```python
from build123d import *


with BuildPart() as part:
    # Sketch1 → Revolve1 (revolve)
    with BuildSketch(Plane.XY):
        with BuildLine():
            Line((0, 0), (0, 7.14024037))
            ThreePointArc((0, 7.14024037), (-10.863552097, 19.485230229), (-24.489599009, 10.279450287))
            ThreePointArc((-24.489599009, 10.279450287), (-27.821731607, 7.348582007), (-31.501935722, 9.82833889))
            ThreePointArc((-31.501935722, 9.82833889), (-35.138176859, 13.576179652), (-40.254364407, 12.530624802))
            ThreePointArc((-40.254364407, 12.530624802), (-42.51580515, 12.328830241), (-44.6786, 13.019593379))
            Line((-44.6786, 13.019593379), (-45.466, 13.019593379))
            Line((-45.466, 13.019593379), (-45.466, 0))
            Line((-45.466, 0), (0, 0))
        make_face()
    revolve(axis=Axis((-45.466, 0, 0), (0, 1, 0)))


solid = part.part
```
CAD build for the part. Positions are in the model's coordinates, mm. Coordinates: 2 decimals unless noted, no trailing zeros. Order: outer loops, then holes, each group sorted by start corner. A loop starts at its lowest first (then second) coordinate and runs counter-clockwise, first axis right, second up. Notation, with made-up numbers: M 42.25,34 L 53.25,34 A31 cw 53.25,61 Z; hole C -28.5,-38 d6. An arc over 180 degrees is marked long. Write each question's results on one line, items separated by ' | '. Start each with the question number.
Q1. Flat gauge pins, fed straight in: P1, Ø8, axis at y = 9.5, z = 33.5, coming from the +X side; P2, Ø6, axis at x = -28, z = 13.5, coming from the +Y side; P3, Ø6, axis at x = -25.5, y = 9.5, coming from the -Z side. Where does each tip first touch, or does it go through?
Q2. Drill centre lines: probe 1 along Z at (x, y) = (-42, 11.5); probe 2 along X at (y, z) = (12.5, -9); probe 3 along Z at (x, y) = (-45, 11.5). Where is each one in solid material? Low to high. Write a range as from..to.
Q3. Cut at A-A (y = 18.25). List the corners of the cut face in (x, z).
Found:
1) P1: x = -11.07 | P2: y = 16.72 | P3: z = -42.03
2) probe 1: -44.54..-21.08, -12.71..12.71, 21.08..44.54 | probe 2: -88.79..-65.31, -53.81..-37.12, -25.62..-2.14 | probe 3: -44.67..-21.36, -13.17..13.17, 21.36..44.67
3) outline: C -45.47,0 d77.26; hole C -45.47,0 d54.82
